from build123d import *

# Parameters (mm, degrees)
SKETCH1_W           = 30
SKETCH1_H           = 25
SKETCH1_R           = 1.5
BOSS_EXTRUDE1_DEPTH = 10
SKETCH3_R           = 4.25
CUT_EXTRUDE1_DEPTH  = 1


with BuildPart() as part:
    # Sketch1 → Boss-Extrude1 (new body)
    with BuildSketch(Plane(origin=(0, 0, 0), x_dir=(1, 0, 0), z_dir=(0, 1, 0))):
        Rectangle(SKETCH1_W, SKETCH1_H)
        with Locations((10, 0)):
            Circle(SKETCH1_R, mode=Mode.SUBTRACT)
        with Locations((-10, 0)):
            Circle(SKETCH1_R, mode=Mode.SUBTRACT)
    extrude(amount=BOSS_EXTRUDE1_DEPTH)

    # Sketch3 → Cut-Extrude1 (cut)
    with BuildSketch(Plane(origin=(0, 10, 0), x_dir=(1, 0, 0), z_dir=(0, 1, 0))):
        Circle(SKETCH3_R)
    extrude(amount=-CUT_EXTRUDE1_DEPTH, mode=Mode.SUBTRACT)


solid = part.part
The listing builds one solid part. Answer for the finished solid, in the listing's coordinates (mm). A direction names the side the tool comes from. Give positions to 0.01 mm unless a question says otherwise; leave off trailing zeros. Write each loop counter-clockwise with the first axis right and the second up, starting at its lowest first coordinate (ties: lowest second). Pieces come first, ordered by that corner, then holes. Notation, with made-up numbers: (40, 61) -> (55, 61) arc R33 cw to (55, 91) -> close; hole circle Ø4 at (44.25, 0). An arc over 180 degrees is marked (long way). Use a Markdown table: item, result.
(1) Section A-A, the plane x = 10 is taken. Determine the outline of the cut face in (y, z), then the cut area to 3 significant figures.
Return value:
| item | result |
|---|---|
| outline | (0, -12.5) -> (10, -12.5) -> (10, -1.5) -> (0, -1.5) -> close; (0, 1.5) -> (10, 1.5) -> (10, 12.5) -> (0, 12.5) -> close |
| area | 220 mm2 |
(2) Section C-C, the plane y = 7 is taken. Determine the outline of the cut face in (x, z).
Return value:
| item | result |
|---|---|
| outline | (-15, -12.5) -> (15, -12.5) -> (15, 12.5) -> (-15, 12.5) -> close; hole circle Ø3 at (-10, 0); hole circle Ø3 at (10, 0) |
(3) Section D-D, the plane x = 2.25 is taken. Determine the outline of the cut face in (y, z).
Return value:
| item | result |
|---|---|
| outline | (0, -12.5) -> (10, -12.5) -> (10, -3.61) -> (9, -3.61) -> (9, 3.61) -> (10, 3.61) -> (10, 12.5) -> (0, 12.5) -> close |
(4) Determine the mould class of faces 1 (the flat face through (0, 0, 0)), 2 (the flat face through (0, 5, 12.5)), 3 (the cylindrical face through (8.5, 4.93, -0.07)) for opening direction Z: released by +Z, released by -Z, zero draft, split by the parting line, or undercut.
Return value:
| item | result |
|---|---|
| face 1 | zero draft |
| face 2 | released by +Z |
| face 3 | undercut |
(5) Section B-B, the plane z = 2 is taken. Determine the outline of the cut face in (x, y), then the cut area to 4 significant figures.
Return value:
| item | result |
|---|---|
| outline | (-15, 0) -> (15, 0) -> (15, 10) -> (3.75, 10) -> (3.75, 9) -> (-3.75, 9) -> (-3.75, 10) -> (-15, 10) -> close |
| area | 292.5 mm2 |
(6) A flat-ended cylindrical pin translates along its axis: P1, Ø2.5, axis at x = 10, z = 0, coming from the -Y side. Find the tip coordinate at first contact, or state that the pin passes through.
Return value:
| item | result |
|---|---|
| P1 | through |
(7) Find the intervals of material crossed by probe 1 along X at (y, z) = (3, 0); probe 2 along Z at (x, y) = (-10, 3); probe 3 along Z at (x, y) = (0, 9.8), in increasing order. Write a range as from..to.
Return value:
| item | result |
|---|---|
| probe 1 | -15..-11.5, -8.5..8.5, 11.5..15 |
| probe 2 | -12.5..-1.5, 1.5..12.5 |
| probe 3 | -12.5..-4.25, 4.25..12.5 |
(8) For faces 4 (the flat face through (0, 9, 0)), 5 (the flat face through (-15, 5, 0)), determine the directions among +Z, -Z, +X, -X, +Y, -Y from which every point of the face is accessible in a straight line to the end or side of a thin tool.
Return value:
| item | result |
|---|---|
| face 4 | +Y |
| face 5 | +Z, -Z, -X, +Y, -Y |
